Verification items for the finished model (mm, model axes). Face numbers are marked on the shaded views. A direction names the side the tool comes from. Round coordinates to 2 decimals unless told otherwise and drop trailing zeros. Loops run counter-clockwise (first coordinate to the right, second up) from the corner with the lowest first, then second, coordinate; pieces in that order, holes last. Notation, with made-up numbers: M 67.5,37.25 L 80.5,37.25 A26 ccw 80.5,51.25 Z; hole C 59.25,45 d9. An arc over 180 degrees is marked long. One line per item, written item: value.
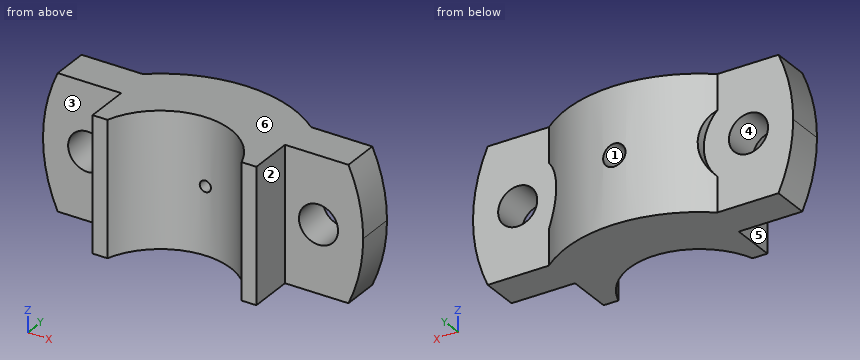
from build123d import *

# Parameters (mm, degrees)
BOSS_EXTRUDE1_DEPTH = 36
CUT_EXTRUDE1_DEPTH  = 10
CUT_EXTRUDE2_DEPTH  = 10
CUT_EXTRUDE8_DEPTH  = 10
SKETCH9_R           = 5.25
CUT_EXTRUDE9_DEPTH  = 10
CUT_EXTRUDE10_DEPTH = 10
SKETCH11_R          = 3
CUT_EXTRUDE11_DEPTH = 10
SKETCH13_R          = 1.5
CUT_EXTRUDE12_DEPTH = 10
FILLET2_R           = 1


with BuildPart() as part:
    # Sketch1 → Boss-Extrude1 (new body)
    with BuildSketch(Plane.XY):
        with BuildLine():
            Line((-22.627416998, 20.226289935), (-43, 20.226289935))
            Line((-43, 20.226289935), (-43, 10.226289935))
            Line((-43, 10.226289935), (-22, 10.226289935))
            Line((-22, 10.226289935), (-22, -1.773710065))
            Line((-22, -1.773710065), (-18.027756377, -1.773710065))
            ThreePointArc((-18.027756377, -1.773710065), (0, 11.226289935), (18.027756377, -1.773710065))
            Line((18.027756377, -1.773710065), (22, -1.773710065))
            Line((22, -1.773710065), (22, 10.226289935))
            Line((22, 10.226289935), (43, 10.226289935))
            Line((43, 10.226289935), (43, 20.226289935))
            Line((43, 20.226289935), (22.627416998, 20.226289935))
            ThreePointArc((22.627416998, 20.226289935), (0, 28.226289935), (-22.627416998, 20.226289935))
        make_face()
    extrude(amount=BOSS_EXTRUDE1_DEPTH)

    # Sketch3 → Cut-Extrude1 (cut)
    with BuildSketch(Plane(origin=(0, 20.226289935, 0), x_dir=(1, 0, 0), z_dir=(0, 1, 0))):
        with BuildLine():
            ThreePointArc((-43, -18), (-42.001212365, -8.785980256), (-39.05124838, 0))
            Line((-39.05124838, 0), (-43, 0))
            Line((-43, 0), (-43, -18))
        make_face()
    extrude(amount=-CUT_EXTRUDE1_DEPTH, mode=Mode.SUBTRACT)

    # Sketch4 → Cut-Extrude2 (cut)
    with BuildSketch(Plane(origin=(0, 20.226289935, 0), x_dir=(1, 0, 0), z_dir=(0, 1, 0))):
        with BuildLine():
            ThreePointArc((-39.05124838, -36), (-42.001212365, -27.214019744), (-43, -18))
            Line((-43, -18), (-43, -36))
            Line((-43, -36), (-39.05124838, -36))
        make_face()
    extrude(amount=-CUT_EXTRUDE2_DEPTH, mode=Mode.SUBTRACT)

    # Sketch5 → Cut-Extrude8 (cut)
    with BuildSketch(Plane(origin=(0, 20.226289935, 0), x_dir=(1, 0, 0), z_dir=(0, 1, 0))):
        with BuildLine():
            Line((43, -36), (43, -18))
            ThreePointArc((43, -18), (42.001212365, -27.214019744), (39.05124838, -36))
            Line((39.05124838, -36), (43, -36))
        make_face()
        with BuildLine():
            ThreePointArc((39.05124838, 0), (42.001212365, -8.785980256), (43, -18))
            Line((43, -18), (43, 0))
            Line((43, 0), (39.05124838, 0))
        make_face()
    extrude(amount=-CUT_EXTRUDE8_DEPTH, mode=Mode.SUBTRACT)

    # Sketch9 → Cut-Extrude9 (cut)
    with BuildSketch(Plane(origin=(0, 20.226289935, 0), x_dir=(1, 0, 0), z_dir=(0, 1, 0))):
        with Locations((31, -18)):
            Circle(SKETCH9_R)
        with Locations((-31, -18)):
            Circle(SKETCH9_R)
    extrude(amount=-CUT_EXTRUDE9_DEPTH, mode=Mode.SUBTRACT)

    # Sketch10 → Cut-Extrude10 (cut)
    with BuildSketch(Plane(origin=(0, 20.226289935, 0), x_dir=(1, 0, 0), z_dir=(0, 1, 0))):
        with BuildLine():
            Line((22.627416998, -9.403497579), (22.627416998, -26.596502421))
            ThreePointArc((22.627416998, -26.596502421), (19, -18), (22.627416998, -9.403497579))
        make_face()
        with BuildLine():
            Line((-22.627416998, -9.403497579), (-22.627416998, -26.596502421))
            ThreePointArc((-22.627416998, -26.596502421), (-19, -18), (-22.627416998, -9.403497579))
        make_face()
    extrude(amount=CUT_EXTRUDE10_DEPTH, mode=Mode.SUBTRACT)

    # Sketch11 → Cut-Extrude11 (cut)
    with BuildSketch(Plane(origin=(0, 28.226289935, 0), x_dir=(1, 0, 0), z_dir=(0, 1, 0))):
        with Locations((0, -18)):
            Circle(SKETCH11_R)
    extrude(amount=-CUT_EXTRUDE11_DEPTH, mode=Mode.SUBTRACT)

    # Sketch13 → Cut-Extrude12 (cut)
    with BuildSketch(Plane(origin=(0, 18.226289935, 0), x_dir=(1, 0, 0), z_dir=(0, 1, 0))):
        with Locations((0, -18)):
            Circle(SKETCH13_R)
    extrude(amount=-CUT_EXTRUDE12_DEPTH, mode=Mode.SUBTRACT)

    # Fillet2
    fillet2_edges = [part.edges().sort_by_distance(p)[0] for p in [
        (-3, 18.226289935, 18),
    ]]
    fillet(fillet2_edges, radius=FILLET2_R)


solid = part.part
(1) Tool access check on the marked faces 1, 2 and 3. Record the directions out of +Z, -Z, +X, -X, +Y, -Y that give a thin tool (end or side, any length) a straight path to the whole face; none if there is none.
Completed:
face 1: +Y
face 2: +Z, -Z, +X, -Y
face 3: +Z, -Z, -X, -Y
(2) Sectioned sample at A-A on x = 0. Enter the section's corners in (y, z).
Completed:
outline: M 11.23,0 L 28.23,0 L 28.23,15 L 19.23,15 A1 cw 18.23,16 L 18.23,16.5 L 11.23,16.5 Z; M 11.23,19.5 L 18.23,19.5 L 18.23,20 A1 cw 19.23,21 L 28.23,21 L 28.23,36 L 11.23,36 Z
(3) Sectioned sample at B-B on y = 13. Enter the section's corners in (x, z), and give its area (3 significant figures).
Completed:
outline: M -39.05,0 L 39.05,0 A43 ccw 39.05,36 L -39.05,36 A43 ccw Z; hole C -31,18 d10.5; hole C 0,18 d3; hole C 31,18 d10.5
area: 2,820 mm^2
(4) Thickness scan on L1, parallel to X at y = 15.75, z = 18; L2, parallel to Z at x = -31, y = 17; L3, parallel to X at y = 3, z = 8. Record the ranges inside material, lowest first. Write a range as from..to.
Completed:
L1: x = -43..-36.25, -25.75..-1.5, 1.5..25.75, 36.25..43
L2: z = 0..12.75, 23.25..36
L3: x = -22..-15.65, 15.65..22
(5) Sectioned sample at D-D on x = 31. Enter the section's corners in (y, z), and give its area (3 significant figures).
Completed:
outline: M 10.23,0 L 20.23,0 L 20.23,12.75 L 10.23,12.75 Z; M 10.23,23.25 L 20.23,23.25 L 20.23,36 L 10.23,36 Z
area: 255 mm^2
(6) Depth check by flat-ended pin: pin 1 Ø12 at (x, z) = (-31.5, 20) entering from +Y; pin 2 Ø13.5 at (x, z) = (31, 18) entering from -Y; pin 3 Ø5 at (x, z) = (0, 18) entering from -Y; pin 4 Ø2.5 at (x, z) = (0, 18) entering from +Y. Enter the tip coordinate at first touch or a pass-through.
Completed:
pin 1: stops at y = 20.23
pin 2: stops at y = 10.23
pin 3: stops at y = 11.06
pin 4: passes through
(7) Sectioned sample at C-C on z = 30. Enter the section's corners in (x, y).
Completed:
outline: M -41.29,10.23 L -22,10.23 L -22,-1.77 L -18.03,-1.77 A19 cw 18.03,-1.77 L 22,-1.77 L 22,10.23 L 41.29,10.23 L 41.29,20.23 L 22.63,20.23 A36 ccw -22.63,20.23 L -41.29,20.23 Z
(8) Mould release check, pull along Z, two halves, no side actions. Record for the marked faces 4, 5 and 6: +Z half, -Z half, draft (parallel to the pull), parting line (faces both ways), or undercut.
Completed:
face 4: undercut
face 5: draft
face 6: +Z half
